from build123d import *

# Parameters (mm, degrees)
SKETCH_1_W        = 12.8
SKETCH_1_H        = 7.3
SKETCH_1_R        = 1
EXTRUDE_1_DEPTH   = 3.2
SKETCH_2_W        = 0.5
SKETCH_2_H        = 3.2
EXTRUDE_1_2_DEPTH = 4
EXTRUDE_2_DEPTH   = 2


with BuildPart() as part:
    # Эскиз1 → Extrude 1 (new, symmetric)
    with BuildSketch(Plane.XY):
        with Locations((-6.4, 3.65)):
            Rectangle(SKETCH_1_W, SKETCH_1_H)
        with Locations((-9.65, 1.5)):
            Circle(SKETCH_1_R, mode=Mode.SUBTRACT)
        with Locations(Location((-3.15, 1.5, 0), (0, 0, 180))):
            Circle(SKETCH_1_R, mode=Mode.SUBTRACT)
    extrude(amount=EXTRUDE_1_DEPTH, both=True)

    # Эскиз2 → Extrude 1 2 (add)
    with BuildSketch(Plane.XZ):
        with Locations((-11.8, 0)):
            Rectangle(SKETCH_2_W, SKETCH_2_H)
        with Locations((-5.874787357, 0)):
            Rectangle(SKETCH_2_W, SKETCH_2_H)
        with Locations((-1, 0)):
            Rectangle(SKETCH_2_W, SKETCH_2_H)
    extrude(amount=EXTRUDE_1_2_DEPTH)

    # Эскиз3 → Вытянуть-Тонкостенный2 (add, symmetric)
    with BuildSketch(Plane.XY):
        Polygon((-12.745952005, 7.055912282), (1.254047995, 10.155912282), (1.145952005, 10.644087718), (-12.854047995, 7.544087718), align=None)
    extrude(amount=EXTRUDE_2_DEPTH, both=True)


solid = part.part
CAD build for the part. Positions are in the model's coordinates, mm. A direction names the side the tool comes from. Round coordinates to 2 decimals unless told otherwise and drop trailing zeros. Loops run counter-clockwise (first coordinate to the right, second up) from the corner with the lowest first, then second, coordinate; pieces in that order, holes last.
(1) Two-plate mould, pull along X, no slides. Class faces 1 (the cylindrical face through (-8.726, 1.117, -0.045)), 2 (the flat face through (-5.756, 9.116, 0.028)), 3 (the flat face through (-5, 9, 2)): +X half, -X half, draft (parallel to the pull), parting line (faces both ways), or undercut.
(2) Cut at C-C (y = 1.5). Give the cut face in (x, z), plus the area to 3 significant figures.
(3) Cut at B-B (z = 0.25). Give the cut face in (x, y).
(4) Which spindle directions (+Z, -Z, +X, -X, +Y, -Y) get a long thin tool onto all of the face, cutting with end or side? Do faces 4 (the flat face through (-6.125, -2, 0)), 5 (the flat face through (-5.285, 8.708, 0.028)), 6 (the flat face through (0, 4, 0)), 7 (the flat face through (-12.8, 4, 0)). Say none if no direction does.
(5) Cut at A-A (y = -1). Give the cut face in (x, z).
(6) Wall check: line 1 along Y through (x, z) = (-9.65, 1.75); line 2 along Y through (x, z) = (-3.15, -1.75); line 3 along X through (y, z) = (2.25, -1). Give the ranges that are in metal, low to high.
(7) Drop flat-ended pins along their axis: pin 1 (3 mm diameter, centred on x = -2.5, z = -2.5, fed in from +Y); pin 2 (1 mm diameter, centred on x = -9.5, z = -1, fed in from +Y); pin 3 (3 mm diameter, centred on x = -9, z = -1, fed in from -Y); pin 4 (1.8 mm diameter, centred on x = -3.15, y = 1.5, fed in from -Z). Give the stop position or say it passes through.
(8) Cut at D-D (z = 2.25). Give the cut face in (x, y), plus the area to 3 significant figures.
Findings below:
1. face 1: undercut
1. face 2: -X half
1. face 3: draft
2. outline: (-12.8, -3.2) - (-10.65, -3.2) - (-10.65, 3.2) - (-12.8, 3.2) - close; (-8.65, -3.2) - (-4.15, -3.2) - (-4.15, 3.2) - (-8.65, 3.2) - close; (-2.15, -3.2) - (0, -3.2) - (0, 3.2) - (-2.15, 3.2) - close
2. area: 56.3 mm2
3. outline: (-12.85, 7.54) - (-12.8, 7.3) - (-12.8, 0) - (-12.05, 0) - (-12.05, -4) - (-11.55, -4) - (-11.55, 0) - (-6.12, 0) - (-6.12, -4) - (-5.62, -4) - (-5.62, 0) - (-1.25, 0) - (-1.25, -4) - (-0.75, -4) - (-0.75, 0) - (0, 0) - (0, 7.3) - (-11.64, 7.3) - (1.25, 10.16) - (1.15, 10.64) - close; hole circle Ø2 at (-9.65, 1.5); hole circle Ø2 at (-3.15, 1.5)
4. face 4: +Z, -Z, -Y
4. face 5: +Z, -Z, +X
4. face 6: +Z, -Z, +X, -Y
4. face 7: +Z, -Z, -X, -Y
5. outline: (-12.05, -1.6) - (-11.55, -1.6) - (-11.55, 1.6) - (-12.05, 1.6) - close; (-6.12, -1.6) - (-5.62, -1.6) - (-5.62, 1.6) - (-6.12, 1.6) - close; (-1.25, -1.6) - (-0.75, -1.6) - (-0.75, 1.6) - (-1.25, 1.6) - close
6. line 1: y = 0 to 0.5, 2.5 to 7.3, 7.74 to 8.25
6. line 2: y = 0 to 0.5, 2.5 to 7.3, 9.18 to 9.69
6. line 3: x = -12.8 to -10.31, -8.99 to -3.81, -2.49 to 0
7. pin 1: stops at y = 10.15
7. pin 2: stops at y = 8.4
7. pin 3: stops at y = 0
7. pin 4: passes through
8. outline: (-12.8, 0) - (0, 0) - (0, 7.3) - (-12.8, 7.3) - close; hole circle Ø2 at (-9.65, 1.5); hole circle Ø2 at (-3.15, 1.5)
8. area: 87.2 mm2
